from build123d import *

# Parameters (mm, degrees)
F1_DEPTH = 584.2
F2_DEPTH = 457.2
F3_DEPTH = 635
F5_DEPTH = 381.001


with BuildPart() as f1:
    # F0 (on Front) → F1 (new body, symmetric)
    with BuildSketch(Plane.XZ):
        Polygon((0, -152.4), (0, 152.4), (-152.4, 152.4), (-1016, 152.4), (-1016, -152.4), (-254, -152.4), align=None)
        Polygon((1016, -152.4), (1016, 152.4), (152.4, 152.4), (0, 152.4), (0, -152.4), (254, -152.4), align=None)
        Polygon((254, -228.6), (254, -152.4), (0, -152.4), (-254, -152.4), (-254, -228.6), align=None)
    extrude(amount=F1_DEPTH, both=True)

    # F0 (on Front) → F2 (join, symmetric)
    with BuildSketch(Plane.XZ):
        with BuildLine():
            Line((-152.4, 152.4), (0, 152.4))
            Line((0, 152.4), (0, 533.4))
            ThreePointArc((0, 533.4), (-77.3134246734, 539.9843385264), (-152.4, 559.5477061887))
            Line((-152.4, 559.5477061887), (-152.4, 152.4))
        make_face()
        with BuildLine():
            Line((0, 152.4), (152.4, 152.4))
            Line((152.4, 152.4), (152.4, 559.5477061887))
            ThreePointArc((152.4, 559.5477061887), (77.3134246734, 539.9843385264), (0, 533.4))
            Line((0, 533.4), (0, 152.4))
        make_face()
    extrude(amount=F2_DEPTH, both=True)

    # F0 (on Front) → F3 (join, symmetric)
    with BuildSketch(Plane.XZ):
        with BuildLine():
            Line((152.4, 685.8), (152.4, 559.5477061887))
            ThreePointArc((152.4, 559.5477061887), (373.3022368002, 726.6354569265), (457.2, 990.6))
            ThreePointArc((457.2, 990.6), (-263.9645430735, 1363.9022368002), (-152.4, 559.5477061887))
            Line((-152.4, 559.5477061887), (-152.4, 685.8))
            Line((-152.4, 685.8), (0, 685.8))
            Line((0, 685.8), (152.4, 685.8))
        make_face()
        with BuildLine():
            ThreePointArc((228.6, 990.6), (161.6446101792, 828.9553898208), (0, 762))
            ThreePointArc((0, 762), (-161.6446101792, 1152.2446101792), (228.6, 990.6))
        make_face(mode=Mode.SUBTRACT)
        with BuildLine():
            ThreePointArc((-152.4, 559.5477061887), (-77.3134246734, 539.9843385264), (0, 533.4))
            Line((0, 533.4), (0, 685.8))
            Line((0, 685.8), (-152.4, 685.8))
            Line((-152.4, 685.8), (-152.4, 559.5477061887))
        make_face()
        with BuildLine():
            ThreePointArc((0, 533.4), (77.3134246734, 539.9843385264), (152.4, 559.5477061887))
            Line((152.4, 559.5477061887), (152.4, 685.8))
            Line((152.4, 685.8), (0, 685.8))
            Line((0, 685.8), (0, 533.4))
        make_face()
    extrude(amount=F3_DEPTH, both=True)

    # F4 (on face) → F5 (cut, through all)
    with BuildSketch(Plane.XY.offset(152.4)):
        Polygon((-812.8, 254), (-812.8, 0), (-812.8, -254), (-558.8, -254), (-558.8, 254), align=None)
        with BuildLine():
            ThreePointArc((-558.8, 254), (-685.8, 381), (-812.8, 254))
            Line((-812.8, 254), (-558.8, 254))
        make_face()
        with BuildLine():
            Line((-558.8, -254), (-812.8, -254))
            ThreePointArc((-812.8, -254), (-685.8, -381), (-558.8, -254))
        make_face()
        Polygon((812.8, -254), (812.8, 0), (812.8, 254), (558.8, 254), (558.8, -254), align=None)
        with BuildLine():
            Line((558.8, 254), (812.8, 254))
            ThreePointArc((812.8, 254), (685.8, 381), (558.8, 254))
        make_face()
        with BuildLine():
            ThreePointArc((558.8, -254), (685.8, -381), (812.8, -254))
            Line((812.8, -254), (558.8, -254))
        make_face()
    extrude(amount=-F5_DEPTH, mode=Mode.SUBTRACT)


solid = f1.part
The model under review builds one solid part; all positions refer to its coordinate system, in mm. A direction names the side the tool comes from. Coordinates: 2 decimals unless noted, no trailing zeros. Loops run counter-clockwise (first coordinate to the right, second up) from the corner with the lowest first, then second, coordinate; pieces in that order, holes last. Notation, with made-up numbers: M -17.5,25.25 L 19.5,25.25 A22 cw 19.5,34.25 Z; hole C 62.5,60.25 d1. An arc over 180 degrees is marked long. Put each result on its own line as item: value. Start each with the question number.
Q1. Clearance check with flat-ended pins moving along their axes: pin 1 (3 mm diameter, centred on y = -197, z = 1259, fed in from -X); pin 2 (5 mm diameter, centred on y = 393.5, z = 286, fed in from -X); pin 3 (23 mm diameter, centred on y = -203.5, z = -186.5, fed in from -X). State where each tip first meets the part, or that it passes through.
Q2. For faces 4 (the flat face through (-14, -584.2, 7)), 5 (the cylindrical face through (688.59, 380.97, 2.13)), 6 (the flat face through (-152.4, -6, 359)), list the 3-axis set-ups (+Z, -Z, +X, -X, +Y, -Y) from which the entire face can be reached by the end or side of a thin tool; tool diameter is ignored.
Q3. Add section B-B (x = 0). Write out the cut boundary in (y, z).
Q4. Add section A-A (y = -505). Write out the cut boundary in (x, z), and give its area (3 significant figures).
Q5. Wall thickness on line 1 (X direction, y = -295.5, z = 990.6); line 2 (Z direction, x = 4, y = 24) (1 decimal); line 3 (Z direction, x = 354, y = -279): over which ranges is each line inside the solid? List them lowest first.
Q6. The part is to be moulded in two halves that separate along Z. For faces 1 (the flat face through (-2, -457.2, 359)), 2 (the flat face through (-254, -8, -190)), 3 (the flat face through (545, -8, -152.4)), say which applies: +Z half, -Z half, draft (parallel to the pull), parting line (faces both ways), or undercut.
Q7. Add section D-D (z = 990.6). Write out the cut boundary in (x, y), and give its area (3 significant figures).
Q8. Add section C-C (y = 215). Write out the cut boundary in (x, z).
Answers:
1. pin 1: stops at x = -371.21
1. pin 2: stops at x = -152.4
1. pin 3: stops at x = -254
2. face 4: -Z, +X, -X, -Y
2. face 5: +Z, -Z
2. face 6: -X, +Y, -Y
3. outline: M -635,533.4 L -457.2,533.4 L -457.2,152.4 L -584.2,152.4 L -584.2,-228.6 L 584.2,-228.6 L 584.2,152.4 L 457.2,152.4 L 457.2,533.4 L 635,533.4 L 635,762 L -635,762 Z; M -635,1219.2 L 635,1219.2 L 635,1447.8 L -635,1447.8 Z
4. outline: M -1016,-152.4 L -254,-152.4 L -254,-228.6 L 254,-228.6 L 254,-152.4 L 1016,-152.4 L 1016,152.4 L -1016,152.4 Z; C 0,990.6 d914.4; hole C 0,990.6 d457.2
4. area: 1,150,000 mm^2
5. line 1: x = -457.2 to -228.6, 228.6 to 457.2
5. line 2: z = -228.6 to 762, 1219.2 to 1447.8
5. line 3: z = -152.4 to 152.4, 701.26 to 1279.94
6. face 1: undercut
6. face 2: draft
6. face 3: -Z half
7. outline: M -457.2,-635 L -228.6,-635 L -228.6,635 L -457.2,635 Z; M 228.6,-635 L 457.2,-635 L 457.2,635 L 228.6,635 Z
7. area: 581,000 mm^2
8. outline: M -1016,-152.4 L -812.8,-152.4 L -812.8,152.4 L -1016,152.4 Z; M -558.8,-152.4 L -254,-152.4 L -254,-228.6 L 254,-228.6 L 254,-152.4 L 558.8,-152.4 L 558.8,152.4 L 152.4,152.4 L 152.4,559.55 A457.2 ccw long -152.4,559.55 L -152.4,152.4 L -558.8,152.4 Z; M 812.8,-152.4 L 1016,-152.4 L 1016,152.4 L 812.8,152.4 Z; hole C 0,990.6 d457.2
